Autodesk Inventor part; units mm, degrees
ref_plane "YZ Plane" through (0, 0, 0) normal (1, 0, 0) x (0, 1, 0)
ref_plane "XZ Plane" through (0, 0, 0) normal (0, 1, 0) x (-1, 0, 0)
ref_plane "XY Plane" through (0, 0, 0) normal (0, 0, 1) x (1, 0, 0)
sketch "Sketch1" plane through (0, 0, 0) normal (0, 0, 1) x (1, 0, 0)
  line L0 (0, 0) -> (88.9, 0)
  line L1 (88.9, 0) -> (88.9, 38.1)
  line L2 (88.9, 38.1) -> (0, 38.1)
  line L3 (0, 38.1) -> (0, 0)
  dimension "d0" = 88.9
  dimension "d1" = 38.1
extrude "Extrusion1" add sketch "Sketch1" along normal blind 101.6
sketch "Sketch3" plane through (0, 38.1, 0) normal (0, 1, 0) x (1, 0, 0)
  line L0 (88.9, 0) -> (0, 0)
  line L1 (88.9, -101.6) -> (0, -101.6)
  line L2 (88.9, 0) -> (88.9, -101.6)
  circle A0 centre (69.85, -50.8) radius 4.3006
  line L3 (44.45, 0) -> (44.45, -101.6) construction
  circle A1 centre (19.05, -50.8) radius 4.3006
  dimension "d4" = 19.05
hole "Hole1" at (19.05, 38.1, 50.8) at (69.85, 38.1, 50.8) direction (0, -1, 0) diameter 5.1054 end through all
sketch "Sketch4" plane through (0, 0, 0) normal (0, -1, 0) x (1, 0, 0)
  circle A0 centre (19.05, 50.8) radius 2.5527
  circle A1 centre (69.85, 50.8) radius 2.5527
  line L0 (0, 0) -> (88.9, 0)
  line L1 (0, 101.6) -> (88.9, 101.6)
  line L2 (44.45, 101.6) -> (44.45, 0) construction
  circle A2 centre (31.75, 69.85) radius 5.9334
  line L3 (19.05, 50.8) -> (69.85, 50.8) construction
  circle A3 centre (57.15, 69.85) radius 5.9334
  point P0 (31.75, 31.75)
  point P1 (57.15, 31.75)
  dimension "d12" = 19.05
  dimension "d13" = 12.7
hole "Hole3" at (31.75, 0, 69.85) at (57.15, 0, 69.85) direction (0, 1, 0) diameter 5.1054 depth 25.4 tip angle 118
properties part number "hubjig_blocks" material "Wood (Cherry)"
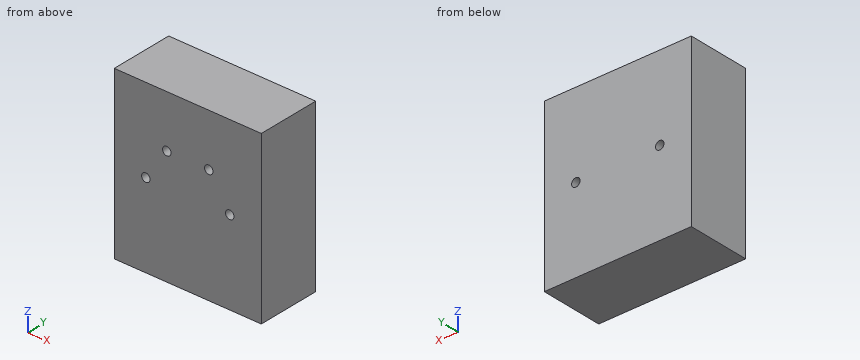
Input: part model. Units: mm. Frame: model coordinates. Coordinates: 2 decimals unless noted, no trailing zeros. Write each loop counter-clockwise with the first axis right and the second up, starting at its lowest first coordinate (ties: lowest second). Pieces come first, ordered by that corner, then holes.
1) Section A-A on x = 69.85. Output: boundary loops of the cut face in (y, z), and give its area (3 significant figures).
2) Pin query (flat end, axial travel): pin 1 Ø4 at (x, z) = (31.75, 69.85) entering from -Y; pin 2 Ø4.5 at (x, z) = (19.05, 50.8) entering from -Y. Return the tip coordinate at first contact, or that it passes through.
3) Material intervals for line 1 along X through (y, z) = (22, 50.8); line 2 along X through (y, z) = (19, 69); line 3 along Z through (x, y) = (31.75, 20), sorted ascending.
Check result:
1. outline: (0, 0) - (38.1, 0) - (38.1, 48.25) - (0, 48.25) - close; (0, 53.35) - (38.1, 53.35) - (38.1, 101.6) - (0, 101.6) - close
1. area: 3,680 mm2
2. pin 1: stops at y = 25.73
2. pin 2: passes through
3. line 1: x = 0 to 16.5, 21.6 to 67.3, 72.4 to 88.9
3. line 2: x = 0 to 29.34, 34.16 to 54.74, 59.56 to 88.9
3. line 3: z = 0 to 67.3, 72.4 to 101.6
